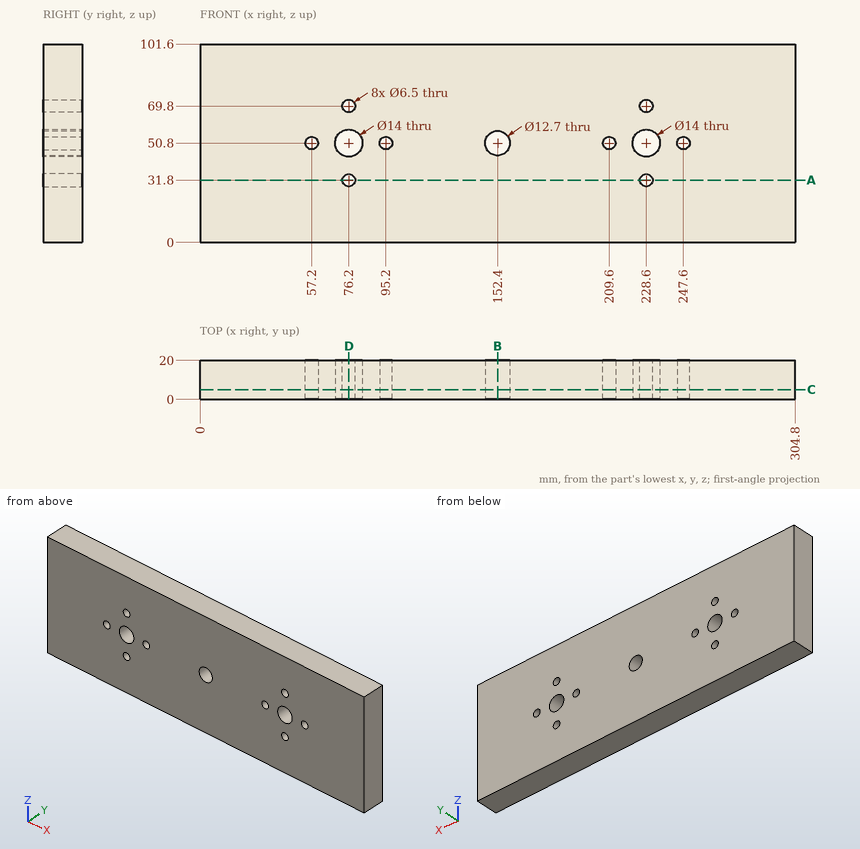
Geometry: see drawing. Coordinates: mm, zero at the bounding-box minimum. Coordinates: 2 decimals unless noted, no trailing zeros. Order: outer loops, then holes, each group sorted by start corner. A loop starts at its lowest first (then second) coordinate and runs counter-clockwise, first axis right, second up. Notation, with made-up numbers: (-17.75, 6) - (40.25, 6) arc R26 ccw to (40.25, 42) - close; hole circle Ø8 at (56, 50). An arc over 180 degrees is marked (long way). Write each question's results on one line, items separated by ' | '.
(1) Line query: line 1 (X direction, y = 15.5, z = 31.8); line 2 (Z direction, x = 209.6, y = 11); line 3 (Z direction, x = 75, y = 14.5). Output: solid intervals per line, ascending. Write a range as [from, to].
Values found:
line 1: x = [0, 72.95], [79.45, 225.35], [231.85, 304.8] | line 2: z = [0, 47.55], [54.05, 101.6] | line 3: z = [0, 28.78], [34.82, 43.9], [57.7, 66.78], [72.82, 101.6]
(2) Section query C-C, the plane y = 5. Count the separate pieces of the cut face and the enclosed holes in it, plus the area to 3 significant figures.
Values found:
separate pieces: 1 | enclosed holes: 11 | area: 30,300 mm²
(3) Section query D-D, the plane x = 76.2. Return the cut outline in (y, z).
Values found:
outline: (0, 0) - (20, 0) - (20, 28.55) - (0, 28.55) - close; (0, 35.05) - (20, 35.05) - (20, 43.8) - (0, 43.8) - close; (0, 57.8) - (20, 57.8) - (20, 66.55) - (0, 66.55) - close; (0, 73.05) - (20, 73.05) - (20, 101.6) - (0, 101.6) - close
(4) Section query B-B, the plane x = 152.4. Return the cut outline in (y, z), plus the area to 3 significant figures.
Values found:
outline: (0, 0) - (20, 0) - (20, 44.45) - (0, 44.45) - close; (0, 57.15) - (20, 57.15) - (20, 101.6) - (0, 101.6) - close | area: 1,780 mm²
(5) Section query A-A, the plane z = 31.8. Return the cut outline in (x, y).
Values found:
outline: (0, 0) - (72.95, 0) - (72.95, 20) - (0, 20) - close; (79.45, 0) - (225.35, 0) - (225.35, 20) - (79.45, 20) - close; (231.85, 0) - (304.8, 0) - (304.8, 20) - (231.85, 20) - close
